from build123d import *

# Parameters (mm, degrees)
ESBO_O1_W                = 157
ESBO_O1_H                = 44.5
RESSALTO_EXTRUS_O1_DEPTH = 14.5
CORTE_EXTRUS_O1_DEPTH    = 0.5
FILETE1_R                = 2


with BuildPart() as part:
    # Esboço1 → Ressalto-extrusão1 (new body, symmetric)
    with BuildSketch(Plane.XY):
        Rectangle(ESBO_O1_W, ESBO_O1_H)
    extrude(amount=RESSALTO_EXTRUS_O1_DEPTH, both=True)

    # Esboço2 → Corte-extrusão1 (cut)
    with BuildSketch(Plane(origin=(78.5, 0, 0), x_dir=(0, 0, -1), z_dir=(1, 0, 0))):
        with BuildLine():
            Line((7.5, 6), (7.5, -6))
            ThreePointArc((7.5, -6), (0, -13.5), (-7.5, -6))
            Line((-7.5, -6), (-7.5, 6))
            ThreePointArc((-7.5, 6), (0, 13.5), (7.5, 6))
        make_face()
    corte_extrus_o1 = extrude(amount=-CORTE_EXTRUS_O1_DEPTH, mode=Mode.SUBTRACT)

    # Espelhar1: Corte-extrusão1 across plane
    add(corte_extrus_o1.mirror(Plane(origin=(0, 0, 0), x_dir=(0, 0, 1), z_dir=(1, 0, 0))), mode=Mode.SUBTRACT)

    # Filete1
    filete1_edges = [part.edges().sort_by_distance(p)[0] for p in [
        (-78.5, 0, 14.5),
        (0, -22.25, 14.5),
        (78.5, 0, 14.5),
        (0, -22.25, -14.5),
        (-78.5, 0, -14.5),
        (0, 22.25, -14.5),
        (78.5, 0, -14.5),
        (0, 22.25, 14.5),
        (78.5, -22.25, 0),
        (-78.5, -22.25, 0),
        (-78.5, 22.25, 0),
        (78.5, 22.25, 0),
    ]]
    fillet(filete1_edges, radius=FILETE1_R)


solid = part.part
Design review of the part built by this model. Coordinates are the model's own, in mm. A direction names the side the tool comes from. Give positions to 0.01 mm unless a question says otherwise; leave off trailing zeros.
1. For pin 1 Ø0.6 at (x, y) = (78, -2.5) entering from -Z; pin 2 Ø1 at (y, z) = (4.5, -4) entering from -X; pin 3 Ø7.5 at (y, z) = (-5.5, -2.5) entering from +X, all flat-tipped, find the tip position at first contact; note any pin that passes through.
Solution:
pin 1: stops at z = -14.1
pin 2: stops at x = -78
pin 3: stops at x = 78
2. To check wall thickness, follow L1, parallel to X at y = 5, z = -6.25; L2, parallel to X at y = -20, z = 12.75; L3, parallel to Y at x = -62, z = -13. State the ranges of each line that lie inside material, in increasing order.
Solution:
L1: x = -78 to 78
L2: x = -78.48 to 78.48
L3: y = -22.19 to 22.19
3. Mouldability with a two-part tool opening along Z and no side actions: class faces 1 (the flat face through (-1, 0, -14.5)), 2 (the cylindrical face through (78.25, 13.5, 0.16)), 3 (the flat face through (-1, 0, 14.5)), 4 (the flat face through (-1, 22.25, 0)) as +Z half, -Z half, draft (parallel to the pull), parting line (faces both ways), or undercut.
Solution:
face 1: -Z half
face 2: undercut
face 3: +Z half
face 4: draft
4. Tool access review of faces 5 (the cylindrical face through (-78.25, 13.5, 0.16)), 6 (the cylindrical face through (78.25, -13.5, -0.16)), 7 (the flat face through (78.5, 0, 9)): name each direction out of +Z, -Z, +X, -X, +Y, -Y from which nothing blocks a thin tool from reaching the whole face with its end or side.
Solution:
face 5: -X
face 6: +X
face 7: +Z, -Z, +X, +Y, -Y
